Read the model definition and answer for the solid it produces. Units are mm, in the model's axes. Face numbers are marked on the shaded views. A direction names the side the tool comes from. Round coordinates to 2 decimals unless told otherwise and drop trailing zeros. Write each loop counter-clockwise with the first axis right and the second up, starting at its lowest first coordinate (ties: lowest second). Pieces come first, ordered by that corner, then holes. Notation, with made-up numbers: (67, 19.5) - (80, 19.5) arc R30 cw to (80, 52.5) - close; hole circle Ø5 at (81, 16). An arc over 180 degrees is marked (long way). One line per item, written item: value. Start each with the question number.
(1) The mould has two halves that part along Y. Classify the marked faces 1, 2 and 3: +Y half, -Y half, draft (parallel to the pull), parting line (faces both ways), or undercut.
(2) Flat-ended cylindrical pins translate along their axes: pin 1 Ø0.8 at (y, z) = (0.5, -0.5) entering from -X; pin 2 Ø8 at (x, z) = (-25, -2) entering from -Y; pin 3 Ø5.5 at (y, z) = (33, 6) entering from +X; pin 4 Ø5 at (y, z) = (40, 4) entering from +X. Find the tip coordinate at first contact, or state that the pin passes through.
(3) Find the intervals of material crossed by L1, parallel to Y at x = -21, z = 5; L2, parallel to Y at x = -12.5, z = 0.25; L3, parallel to Y at x = -24, z = -4.75, in increasing order.
(4) A cutting plane is placed at D-D, the plane y = 5. Determine the outline of the cut face in (x, z), plus the area to 3 significant figures.
(5) A cutting plane is placed at A-A, the plane y = 15.5. Determine the outline of the cut face in (x, z).
(6) A cutting plane is placed at B-B, the plane z = 0. Determine the outline of the cut face in (x, y).
(7) A cutting plane is placed at C-C, the plane z = 6.75. Determine the outline of the cut face in (x, y).
(8) For the marked faces 4, 5 and 6, determine the directions among +Z, -Z, +X, -X, +Y, -Y from which every point of the face is accessible in a straight line to the end or side of a thin tool.
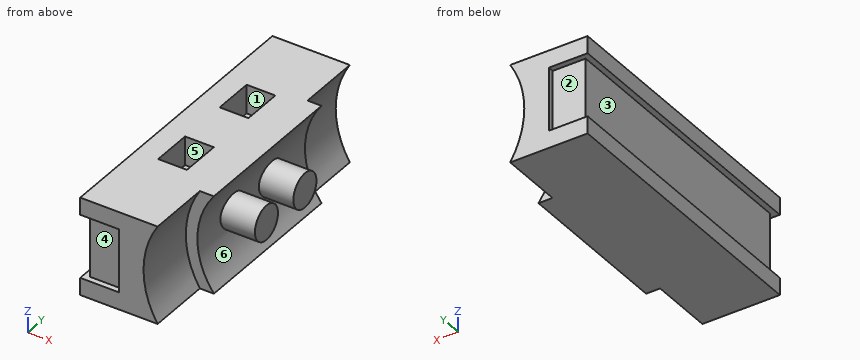
Autodesk Inventor part; units mm, degrees
ref_plane "Work Plane1" through (0, 11, 0) normal (0, -1, 0) x (1, 0, 0)
ref_plane "Work Plane2" through (-13.5554, 11, 8.5) normal (-1, 0, 0) x (0, 1, 0)
ref_plane "Work Plane3" through (0, 39, 0) normal (0, 1, 0) x (1, 0, 0)
sketch "Sketch1" plane through (0, 0, 0) normal (0, 1, 0) x (-1, 0, 0)
  circle A0 centre (0, 0) radius 14
  line L0 (14, 0) -> (27, 0)
  circle A1 centre (0, 0) radius 16
  line L1 (27, 0) -> (27, -8.5)
  line L2 (27, -8.5) -> (13.5552, -8.5)
  line L3 (13.5552, 8.5) -> (27, 8.5)
  line L4 (27, 8.5) -> (27, -8.5)
  line L5 (13.5552, 8.5) -> (11.1243, 8.5)
  line L6 (13.5552, -8.5) -> (11.1243, -8.5)
  line L7 (13.5552, 8.5) -> (13.5552, -8.5)
  dimension "d0" = 28
  dimension "d1" = 13
  dimension "d2" = 32
  dimension "d3" = 8.5
  dimension "d5" = 17
extrude "Extrusion1" add sketch "Sketch1" along normal blind 50 contours L5 L7 A0 | A0 L7 L6 | L7 A1 L0 A0 | L3 L4 L0 A1 | A0 L0 A1 L7 | A1 L0 L1 L2
ref_plane "Work Plane1" through (0, 11, 0) normal (0, -1, 0) x (1, 0, 0)
sketch "Sketch2" plane through (0, 11, 0) normal (0, -1, 0) x (1, 0, 0)
  circle A0 centre (0, 0) radius 16
  line L0 (-11.1243, -8.5) -> (-27, -8.5)
  circle A1 centre (0, 0) radius 14
  line L1 (-27, 8.5) -> (-11.1243, 8.5)
  line L2 (-13.5554, 8.5) -> (-11.1243, 8.5)
  line L3 (-13.5554, -8.5) -> (-11.1243, -8.5)
  dimension "d9" = 32
extrude "Extrusion2" cut sketch "Sketch2" against normal blind 28 contours L1 A1 L0 A0 picked at (-13.7856, -6.5585)
ref_plane "Work Plane2" through (-13.5554, 11, 8.5) normal (-1, 0, 0) x (0, 1, 0)
sketch "Sketch3" plane through (-13.5554, 11, 8.5) normal (-1, 0, 0) x (0, 1, 0)
  line L0 (28, 17) -> (28, 0) construction
  line L1 (28, 8.5) -> (0, 8.5) construction
  line L2 (0, 17) -> (0, 0) construction
  line L3 (28, 8.5) -> (19, 8.5)
  circle A0 centre (19, 8.5) radius 3
  line L4 (0, 8.5) -> (9, 8.5)
  circle A1 centre (9, 8.5) radius 3
  point P0 (-11, 8.5)
  dimension "d14" = 9
  dimension "d15" = 6
  dimension "d17" = 9
  dimension "d18" = 6
extrude "Extrusion3" add sketch "Sketch3" along normal up to surface
sketch "Sketch4" plane through (-13.5554, 30, 0) normal (1, 0, 0) x (0, 0, -1)
  circle A0 centre (0, 0) radius 3
  circle A1 centre (0, 0) radius 3
  point P0 (0, -30)
sketch "Sketch5" plane through (-13.5554, 20, 0) normal (1, 0, 0) x (0, 0, -1)
  circle A0 centre (0, 0) radius 3
  point P0 (0, -20)
extrude "Extrusion4" cut sketch "Sketch4" against normal blind 0.445
extrude "Extrusion5" cut sketch "Sketch5" against normal blind 0.445
sketch "Sketch6" plane through (-14.0004, 30, 0) normal (1, 0, 0) x (0, 0, -1)
  circle A0 centre (0, 0) radius 3
  point P0 (0, -30)
sketch "Sketch7" plane through (-14.0004, 20, 0) normal (1, 0, 0) x (0, 0, -1)
  circle A0 centre (0, 0) radius 3
  point P0 (0, -20)
extrude "Extrusion6" add sketch "Sketch6" along normal blind 6
extrude "Extrusion7" add sketch "Sketch7" along normal up to surface (6 mm away)
sketch "Sketch8" plane through (0, 11, 0) normal (0, 1, 0) x (1, 0, 0)
  circle A0 centre (0, 0) radius 14
  circle A1 centre (0, 0) radius 16
  line L0 (-13.5554, 8.5) -> (-11.1243, 8.5)
  line L1 (-13.5554, 8.5) -> (-11.1243, 8.5)
  arc A2 (-11.1243, 8.5) -> (-11.1243, -8.5) centre (0, 0) ccw
  line L2 (-13.5554, -8.5) -> (-11.1243, -8.5)
  dimension "d29" = 32
sketch "Sketch9" plane through (0, 11, 0) normal (0, 1, 0) x (1, 0, 0)
  circle A0 centre (0, 0) radius 16
  circle A1 centre (0, 0) radius 14
  dimension "d30" = 32
extrude "Extrusion8" add sketch "Sketch8" along normal up to surface (28 mm away) contours A0 L2 A1 L0 picked at (-13.7856, -6.5585)
extrude "Extrusion9" cut sketch "Sketch9" against normal up to surface (11 mm away)
ref_plane "Work Plane3" through (0, 39, 0) normal (0, 1, 0) x (1, 0, 0)
sketch "Sketch10" plane through (0, 39, 0) normal (0, 1, 0) x (1, 0, 0)
  circle A0 centre (0, 0) radius 16
  circle A1 centre (0, 0) radius 14
  dimension "d36" = 32
  dimension "d37" = 28
extrude "Extrusion10" cut sketch "Sketch10" along normal up to surface (11 mm away)
sketch "Sketch11" plane through (-27, 0, -8.5) normal (-1, 0, 0) x (0, 0, 1)
  line L0 (17, 0) -> (17, 50)
  line L1 (17, 50) -> (14, 50)
  line L2 (0, 50) -> (17, 50)
  line L3 (14, 50) -> (3, 50)
  line L4 (0, 0) -> (0, 50)
  line L5 (0, 0) -> (3, 0)
  line L6 (17, 0) -> (0, 0)
  line L7 (14, 50) -> (3, 50)
  line L8 (3, 50) -> (3, 0)
  line L9 (3, 0) -> (14, 0)
  line L10 (14, 0) -> (14, 50)
  point P0 (8.5, 0)
  dimension "d40" = 3
  dimension "d41" = 11
  dimension "d42" = 3
extrude "Extrusion11" cut sketch "Sketch11" against normal blind 1 contours L6 L8 L2 L10
sketch "Sketch12" plane through (0, 50, 0) normal (0, 1, 0) x (1, 0, 0)
  line L0 (-27, -5.5) -> (-27, -8.5)
  line L1 (-27, -5.5) -> (-20.278, -5.5)
  line L2 (-27, 5.5) -> (-26, 5.5)
  line L3 (-20.278, -5.5) -> (-27, -5.5)
  line L4 (-27, -5.5) -> (-27, 5.5)
  line L5 (-27, 5.5) -> (-20.278, 5.5)
  line L6 (-20.278, 5.5) -> (-20.278, -5.5)
  point P0 (0, 0)
  dimension "d45" = 6.722
sketch "Sketch13" plane through (0, 0, 0) normal (0, -1, 0) x (1, 0, 0)
  line L0 (-27, -5.5) -> (-26, -5.5)
  line L1 (-27, -5.5) -> (-20.278, -5.5)
  line L2 (-20.278, -5.5) -> (-27, -5.5)
  line L3 (-27, -5.5) -> (-27, 5.5)
  line L4 (-27, 5.5) -> (-20.278, 5.5)
  line L5 (-20.278, 5.5) -> (-20.278, -5.5)
  point P0 (0, 0)
  dimension "d46" = 6.722
extrude "Extrusion12" cut sketch "Sketch13" against normal blind 1
extrude "Extrusion13" cut sketch "Sketch12" against normal blind 1
sketch "Sketch14" plane through (-27, 0, 8.5) normal (0, 0, 1) x (1, 0, 0)
  line L0 (0, 50) -> (6.722, 50) construction
  line L1 (6.722, 50) -> (6.722, 41) construction
  line L2 (6.722, 41) -> (6.722, 34) construction
  line L3 (0, 34) -> (0, 31) construction
  line L4 (0, 31) -> (3.361, 31) construction
  line L5 (6.722, 34) -> (3.361, 34) construction
  line L6 (3.361, 34) -> (3.361, 31) construction
  line L7 (3.361, 31) -> (4.861, 31) construction
  line L8 (0, 0) -> (0, 50) construction
  line L9 (4.861, 31) -> (4.861, 38.2796) construction
  line L10 (4.861, 31) -> (7.861, 31) construction
  line L11 (13, 39) -> (13, 11) construction
  line L12 (6.361, 31) -> (6.361, 37.5) construction
  line L13 (4.861, 36.5) -> (7.861, 36.5) construction
  line L14 (7.861, 36.5) -> (7.861, 31.5) construction
  line L15 (7.861, 31.5) -> (4.861, 31.5) construction
  line L16 (4.861, 31.5) -> (4.861, 36.5) construction
  line L17 (4.861, 36.5) -> (7.861, 31.5) construction
  line L18 (7.861, 36.5) -> (4.861, 31.5) construction
  line L19 (6.361, 31.5) -> (6.361, 20.5) construction
  line L20 (6.361, 20.5) -> (6.361, 18) construction
  line L21 (4.861, 15.5) -> (7.861, 15.5) construction
  line L22 (7.861, 15.5) -> (7.861, 20.5) construction
  line L23 (7.861, 20.5) -> (4.861, 20.5) construction
  line L24 (4.861, 20.5) -> (4.861, 15.5) construction
  line L25 (4.861, 15.5) -> (7.861, 20.5) construction
  line L26 (7.861, 15.5) -> (4.861, 20.5) construction
  line L27 (8.861, 21.5) -> (8.861, 14.5)
  line L28 (8.861, 14.5) -> (3.861, 14.5)
  line L29 (3.861, 14.5) -> (3.861, 21.5)
  line L30 (3.861, 21.5) -> (8.861, 21.5)
  line L31 (8.861, 37.5) -> (3.861, 37.5)
  line L32 (3.861, 37.5) -> (3.861, 30.5)
  line L33 (3.861, 30.5) -> (8.861, 30.5)
  line L34 (8.861, 30.5) -> (8.861, 37.5)
  point P0 (27, 0)
  point P1 (6.361, 34)
  dimension "d51" = 9
  dimension "d52" = 7
  dimension "d53" = 3
  dimension "d54" = 1.5
  dimension "d55" = 3
  dimension "d56" = 3
  dimension "d57" = 5
  dimension "d58" = 11
  dimension "d59" = 2.5
  dimension "d60" = 1
  dimension "d61" = 1
extrude "Extrusion14" cut sketch "Sketch14" against normal blind 5
properties part number "Button"
Here are the results:
1. face 1: undercut
1. face 2: +Y half
1. face 3: draft
2. pin 1: x = -20.28
2. pin 2: y = 0
2. pin 3: x = -11.12
2. pin 4: x = -12.51
3. L1: 1 to 14.5, 21.5 to 30.5, 37.5 to 49
3. L2: 17.01 to 22.99, 27.01 to 32.99
3. L3: 1 to 49
4. outline: (-27, -8.5) - (-13.56, -8.5) arc R16 cw to (-13.56, 8.5) - (-27, 8.5) - (-27, 5.5) - (-26, 5.5) - (-26, -5.5) - (-27, -5.5) - close
4. area: 189 mm²
5. outline: (-27, -8.5) - (-11.12, -8.5) arc R14 cw to (-11.12, 8.5) - (-18.14, 8.5) - (-18.14, 3.5) - (-23.14, 3.5) - (-23.14, 8.5) - (-27, 8.5) - (-27, 5.5) - (-26, 5.5) - (-26, -5.5) - (-27, -5.5) - close
6. outline: (-26, 1) - (-20.28, 1) - (-20.28, 0) - (-16, 0) - (-16, 11) - (-14, 11) - (-14, 17) - (-8, 17) - (-8, 23) - (-14, 23) - (-14, 27) - (-8, 27) - (-8, 33) - (-14, 33) - (-14, 39) - (-16, 39) - (-16, 50) - (-20.28, 50) - (-20.28, 49) - (-26, 49) - close
7. outline: (-27, 0) - (-14.51, 0) - (-14.51, 11) - (-12.27, 11) - (-12.27, 39) - (-14.51, 39) - (-14.51, 50) - (-27, 50) - close; hole (-23.14, 14.5) - (-18.14, 14.5) - (-18.14, 21.5) - (-23.14, 21.5) - close; hole (-23.14, 30.5) - (-18.14, 30.5) - (-18.14, 37.5) - (-23.14, 37.5) - close
8. face 4: -X, -Y
8. face 5: +Z
8. face 6: +X
